Work out the finished part from the listing and answer in its coordinate system (mm). Face numbers are marked on the shaded views. A direction names the side the tool comes from. Give positions to 0.01 mm unless a question says otherwise; leave off trailing zeros. Loops run counter-clockwise (first coordinate to the right, second up) from the corner with the lowest first, then second, coordinate; pieces in that order, holes last.
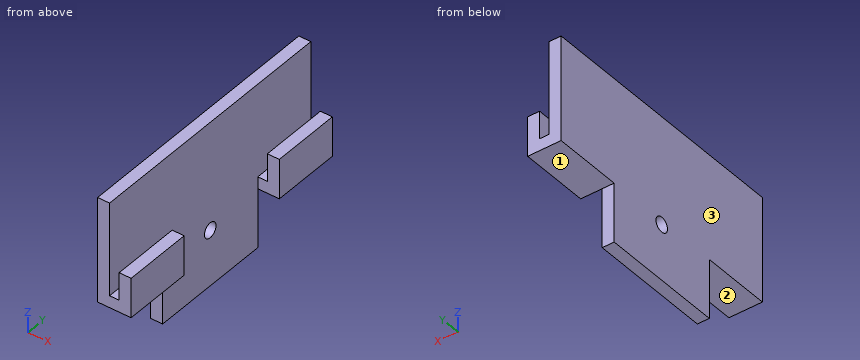
Autodesk Inventor part; units mm, degrees
ref_plane "YZ Plane" through (0, 0, 0) normal (1, 0, 0) x (0, 1, 0)
ref_plane "XZ Plane" through (0, 0, 0) normal (0, 1, 0) x (-1, 0, 0)
ref_plane "XY Plane" through (0, 0, 0) normal (0, 0, 1) x (1, 0, 0)
sketch "Sketch1" plane through (0, 0, 0) normal (0, 1, 0) x (-1, 0, 0)
  line L0 (0, 27.1) -> (0, -27.1)
  line L1 (0, 27.1) -> (-6.8, 27.1)
  line L2 (-6.8, 27.1) -> (-6.8, 18.8)
  line L3 (-6.8, 18.8) -> (-4.3, 18.8)
  line L4 (-4.3, 18.8) -> (-4.3, 24.6)
  line L5 (-4.3, 24.6) -> (-2.5, 24.6)
  line L6 (-2.5, 24.6) -> (-2.5, 0)
  line L7 (0, -27.1) -> (-7, -27.1)
  line L8 (-7, -27.1) -> (-7, -18.8)
  line L9 (-7, -18.8) -> (-4.5, -18.8)
  line L10 (-4.5, -18.8) -> (-4.5, -24.6)
  line L11 (-4.5, -24.6) -> (-2.5, -24.6)
  line L12 (-2.5, -24.6) -> (-2.5, 0)
  point P0 (0, 0)
  dimension "d0" = 54.2
  dimension "d1" = 6.8
  dimension "d2" = 8.3
  dimension "d3" = 2.5
  dimension "d4" = 5.8
  dimension "d5" = 1.8
  dimension "d6" = 8.3
  dimension "d7" = 5.8
extrude "Extrusion1" add sketch "Sketch1" along normal blind 14.5
sketch "Sketch2" plane through (0, 14.5, 0) normal (0, 1, 0) x (1, 0, 0)
  line L0 (2.5, -24.6) -> (2.5, 24.6)
  line L1 (2.5, 0) -> (2.5, 39.5)
  line L2 (2.5, 39.5) -> (0, 39.5)
  line L3 (0, 39.5) -> (0, 0)
  line L4 (0, 0) -> (0, -39.5)
  line L5 (0, 27.1) -> (0, -27.1)
  line L6 (0, -39.5) -> (2.5, -39.5)
  line L7 (2.5, -39.5) -> (2.5, 0)
  point P0 (2.5, -24.6)
  point P1 (2.5, 24.6)
  dimension "d10" = 39.5
  dimension "d11" = 39.5
extrude "Extrusion2" add sketch "Sketch2" along normal blind 26
sketch "Sketch3" plane through (0, 40.5, 0) normal (0, 1, 0) x (1, 0, 0)
  line L0 (2.5, -24.6) -> (2.5, 24.6)
  line L1 (2.5, 0) -> (2.5, 24.6558)
  line L2 (0, 27.1) -> (0, -27.1)
  line L3 (4.3, -24.6) -> (2.5, -24.6)
  line L4 (6.8, -18.8) -> (4.3, -18.8)
  line L5 (4.3, -24.6) -> (4.3, -18.8)
  line L6 (4.3, -18.8) -> (6.8, -18.8)
  line L7 (6.8, -18.8) -> (6.8, -27.1)
  line L8 (6.8, -27.1) -> (2.5, -27.1)
  line L9 (2.5, 0) -> (2.5, 24.6558)
  line L10 (2.5, 24.6) -> (4.5, 24.6)
  line L11 (4.5, 18.8) -> (7, 18.8)
  line L12 (4.5, 24.6) -> (4.5, 18.8)
  line L13 (4.5, 18.8) -> (7, 18.8)
  line L14 (7, 18.8) -> (7, 27.1)
  line L15 (7, 27.1) -> (0, 27.1)
  line L16 (0, 27.1) -> (0, -27.1)
  line L17 (6.8, -27.1) -> (0, -27.1)
  line L18 (4.3, -24.6) -> (2.5, -24.6)
  point P0 (0, 0)
extrude "Extrusion3" add sketch "Sketch3" along normal blind 14.5
sketch "Sketch4" plane through (2.5, 0, 24.6) normal (1, 0, 0) x (0, 0, -1)
  line L0 (64.1, 14.5) -> (64.1, 40.5)
  line L1 (-14.9, 14.5) -> (-14.9, 40.5)
  line L2 (-14.9, 27.5) -> (-1.5, 27.5)
  circle A0 centre (-1.5, 27.5) radius 1.5
  line L3 (64.1, 14.5) -> (64.1, 40.5)
  circle A1 centre (52.4, 27.5) radius 1.575
  line L4 (52.4, 27.5) -> (64.1, 27.5)
  point P0 (24.6, 0)
  dimension "d18" = 13.4
  dimension "d19" = 3
extrude "Extrusion4" cut sketch "Sketch4" against normal blind 4.5
sketch "Sketch5" plane through (0, 0, -27.1) normal (-1, 0, 0) x (0, 0, 1)
  line L0 (27.1, 0) -> (21.3, 0)
  line L1 (51.7, 0) -> (2.5, 0)
  line L2 (21.3, 0) -> (21.3, 55)
  line L3 (51.7, 55) -> (2.5, 55)
  line L4 (27.1, 55) -> (32.9, 55)
  line L5 (32.9, 55) -> (32.9, 0)
  line L6 (32.9, 0) -> (27.1, 0)
  dimension "d22" = 5.8
  dimension "d23" = 5.8
extrude "Extrusion5" cut sketch "Sketch5" against normal blind 62.3875
sketch "Sketch6" plane through (0, 0, 5.8) normal (0, 0, -1) x (-1, 0, 0)
  point P0 (0, 0)
sketch "Sketch7" plane through (0, 14.5, 27.1) normal (-1, 0, 0) x (0, 0, 1)
  line L0 (-21.3, -14.5) -> (0, -14.5)
  line L1 (-21.3, -14.5) -> (18.5957, -14.5)
  line L2 (18.5957, -14.5) -> (18.5957, 49.9868)
  line L3 (18.5957, 49.9868) -> (-21.3, 49.9868)
  line L4 (-21.3, 49.9868) -> (-21.3, -14.5)
  point P0 (-27.1, -14.5)
extrude "Extrusion6" cut sketch "Sketch7" against normal blind 62.3875
sketch "Sketch8" plane through (0, 0, -5.8) normal (0, 0, 1) x (1, 0, 0)
  line L0 (0, 55) -> (2.5, 55)
  line L1 (2.5, 0) -> (0, 0)
  line L2 (2.5, 55) -> (2.5, 0)
  line L3 (2.5, 0) -> (0, 0)
  line L4 (0, 0) -> (0, 55)
extrude "Extrusion7" add sketch "Sketch8" along normal blind 0.7
properties part number "cam_holder3"
Item 1: Flat-ended cylindrical pins translate along their axes: pin 1 Ø12 at (y, z) = (34.5, -34) entering from -X; pin 2 Ø2 at (x, y) = (3.5, 46) entering from -Z; pin 3 Ø0.8 at (x, y) = (6, 44) entering from +Z; pin 4 Ø2 at (x, z) = (1, -33.5) entering from +Y. Find the tip coordinate at first contact, or state that the pin passes through.
Item 2: Consider line 1 (Y direction, x = 1.6, z = -27.8) (3 decimals); line 2 (Z direction, x = 5.75, y = 10); line 3 (X direction, y = 25, z = -34). Determine where each line is inside the solid, lowest interval first.
Item 3: For the marked faces 1, 2 and 3, determine the directions among +Z, -Z, +X, -X, +Y, -Y from which every point of the face is accessible in a straight line to the end or side of a thin tool.
Item 4: Find section A-A, the plane z = -27.8. Write down the section's boundary in (x, y) (3 decimals), plus the area to 3 significant figures.
Item 5: Find section D-D, the plane y = 47. Write down the section's boundary in (x, z), plus the area to 4 significant figures.
Item 6: Find section C-C, the plane z = -20. Write down the section's boundary in (x, y).
Item 7: Find section B-B, the plane y = 27.5. Write down the section's boundary in (x, z) (3 decimals).
Ans:
1. pin 1: stops at x = 0
1. pin 2: stops at z = -27.1
1. pin 3: stops at z = -18.8
1. pin 4: stops at y = 40.5
2. line 1: y = 14.5 to 25.925, 29.075 to 40.5
2. line 2: z = -27.1 to -18.8
2. line 3: x = 0 to 2.5
3. face 1: -Z, +X, -X, +Y
3. face 2: -Z, +X, -X, -Y
3. face 3: +Z, -Z, -X, +Y, -Y
4. outline: (0, 14.5) - (2.5, 14.5) - (2.5, 25.925) - (0, 25.925) - close; (0, 29.075) - (2.5, 29.075) - (2.5, 40.5) - (0, 40.5) - close
4. area: 57.1 mm2
5. outline: (0, -27.1) - (7, -27.1) - (7, -18.8) - (4.5, -18.8) - (4.5, -24.6) - (2.5, -24.6) - (2.5, -5.1) - (0, -5.1) - close
5. area: 80.75 mm2
6. outline: (0, 0) - (2.5, 0) - (2.5, 55) - (0, 55) - close; (4.5, 0) - (7, 0) - (7, 14.5) - (4.5, 14.5) - close; (4.5, 40.5) - (7, 40.5) - (7, 55) - (4.5, 55) - close
7. outline: (0, -39.5) - (2.5, -39.5) - (2.5, -29.375) - (0, -29.375) - close; (0, -26.225) - (2.5, -26.225) - (2.5, -5.1) - (0, -5.1) - close
